Here's how the part is built. I have some questions about the finished solid (model axes, mm). A direction names the side the tool comes from. Give positions to 0.01 mm unless a question says otherwise; leave off trailing zeros. Order: outer loops, then holes, each group sorted by start corner. A loop starts at its lowest first (then second) coordinate and runs counter-clockwise, first axis right, second up.
Autodesk Inventor part; units mm, degrees
ref_plane "YZ Plane" through (0, 0, 0) normal (1, 0, 0) x (0, 1, 0)
ref_plane "XZ Plane" through (0, 0, 0) normal (0, 1, 0) x (-1, 0, 0)
ref_plane "XY Plane" through (0, 0, 0) normal (0, 0, 1) x (1, 0, 0)
sketch "Sketch1" plane through (0, 0, 0) normal (0, 0, 1) x (1, 0, 0)
  circle A0 centre (0, 0) radius 23
  dimension "d0" = 46
extrude "Extrusion1" add sketch "Sketch1" along normal mid plane 6
sketch "Sketch2" plane through (0, 0, 3) normal (0, 0, 1) x (1, 0, 0)
  circle A0 centre (0, 17) radius 1.5
  circle A1 centre (-14.7224, -8.5) radius 1.5
  circle A2 centre (14.7224, -8.5) radius 1.5
  point P0 (0, 0)
  dimension "d3" = 3
  dimension "d4" = 17
  dimension "d7" = 360
hole "Hole1" at (0, 17, 3) at (-14.7224, -8.5, 3) at (14.7224, -8.5, 3) direction (0, 0, -1) diameter 3 end through all counterbore diameter 6 counterbore depth 3
sketch "Sketch3" plane through (0, 0, 3) normal (0, 0, 1) x (1, 0, 0)
  circle A0 centre (0, 0) radius 6
  dimension "d16" = 12
hole "Hole2" at (0, 0, 3) direction (0, 0, -1) diameter 10.106 depth 6
equation "\"d9\" = d3"
properties part number "Gripper_Central_Plate_Base" material "Aluminum 6061"
Q1. I need wall thicknesses on L1, parallel to Y at x = 0, z = 1.7; L2, parallel to Y at x = 0, z = -2.4; L3, parallel to X at y = -8.5, z = -1.9. Which ranges of each line are inside material? Lowest first, please.
Filled sheet:
L1: y = -23 to -5.05, 5.05 to 14, 20 to 23
L2: y = -23 to -5.05, 5.05 to 15.5, 18.5 to 23
L3: x = -21.37 to -16.22, -13.22 to 13.22, 16.22 to 21.37
Q2. If we section it at C-C on x = 15.5: List the corners of the cut face in (y, z) for me, plus the area to 3 significant figures.
Filled sheet:
outline: (-16.99, -3) - (-9.78, -3) - (-9.78, 0) - (-11.4, 0) - (-11.4, 3) - (-16.99, 3) - close; (-7.22, -3) - (16.99, -3) - (16.99, 3) - (-5.6, 3) - (-5.6, 0) - (-7.22, 0) - close
area: 179 mm2
Q3. If we section it at B-B on x = 0: List the corners of the cut face in (y, z) for me, plus the area to 3 significant figures.
Filled sheet:
outline: (-23, -3) - (-5.05, -3) - (-5.05, 3) - (-23, 3) - close; (5.05, -3) - (15.5, -3) - (15.5, 0) - (14, 0) - (14, 3) - (5.05, 3) - close; (18.5, -3) - (23, -3) - (23, 3) - (20, 3) - (20, 0) - (18.5, 0) - close
area: 188 mm2
Q4. If we section it at A-A on y = 0: List the corners of the cut face in (x, z) for me.
Filled sheet:
outline: (-23, -3) - (-5.05, -3) - (-5.05, 3) - (-23, 3) - close; (5.05, -3) - (23, -3) - (23, 3) - (5.05, 3) - close
Q5. I'm going to push flat-ended pins straight in: P1, Ø1.8, axis at x = -16, y = -8.5, coming from the +Z side; P2, Ø2.5, axis at x = 0, y = 17, coming from the -Z side. Where does each tip first touch, or does it pass through?
Filled sheet:
P1: stops at z = 0
P2: passes through
Q6. For faces 1 (the face through (0, 20, 1)), 2 (the face through (13.235, -8.305, -1.521)), which set-ups out of +Z, -Z, +X, -X, +Y, -Y let a thin tool reach every point of the face, with its end or its side?
Filled sheet:
face 1: +Z
face 2: +Z, -Z
Q7. If we section it at D-D on y = -8.5: List the corners of the cut face in (x, z) for me, plus the area to 3 significant figures.
Filled sheet:
outline: (-21.37, -3) - (-16.22, -3) - (-16.22, 0) - (-17.72, 0) - (-17.72, 3) - (-21.37, 3) - close; (-13.22, -3) - (13.22, -3) - (13.22, 0) - (11.72, 0) - (11.72, 3) - (-11.72, 3) - (-11.72, 0) - (-13.22, 0) - close; (16.22, -3) - (21.37, -3) - (21.37, 3) - (17.72, 3) - (17.72, 0) - (16.22, 0) - close
area: 202 mm2
Q8. Thinking about a two-plate mould opening in Y: for faces 3 (the face through (-5.4, 0.3, -3)), 4 (the face through (-2.994, 22.804, 0.042)), 5 (the face through (-14, -7, 0)), which applies, released by +Y, released by -Y, zero draft, split by the parting line, or undercut?
Filled sheet:
face 3: zero draft
face 4: split by the parting line
face 5: undercut
